Source: CAD feature listing. Evaluate the final solid. Frame: model axes, mm. A direction names the side the tool comes from. Round coordinates to 2 decimals unless told otherwise and drop trailing zeros. Write each loop counter-clockwise with the first axis right and the second up, starting at its lowest first coordinate (ties: lowest second). Pieces come first, ordered by that corner, then holes.
```python
from build123d import *

# Parameters (mm, degrees)
SKETCH_1_W          = 15
SKETCH_1_H          = 32
EXTRUDE_1_DEPTH     = 2
SKETCH_2_W          = 10
SKETCH_2_H          = 6
EXTRUDE_2_DEPTH     = 6
CHAMFER_1_SIZE      = 1
SKETCH_3_R          = 1.5
CUT_EXTRUDE_1_DEPTH = 28


with BuildPart() as part:
    # 草图1 → 凸台-拉伸1 (new body)
    with BuildSketch(Plane.XY):
        Rectangle(SKETCH_1_W, SKETCH_1_H)
    extrude(amount=EXTRUDE_1_DEPTH)

    # 草图2 → 凸台-拉伸2 (add)
    with BuildSketch(Plane(origin=(0, 0, 0), x_dir=(-1, 0, 0), z_dir=(0, 0, -1))):
        with Locations((0, 13)):
            Rectangle(SKETCH_2_W, SKETCH_2_H)
    extrude(amount=EXTRUDE_2_DEPTH)

    # 倒角1
    chamfer_1_edges = [part.edges().sort_by_distance(p)[0] for p in [
        (0, 10, -6),
        (-5, 13, -6),
        (0, 16, -6),
        (5, 13, -6),
    ]]
    chamfer(chamfer_1_edges, length=CHAMFER_1_SIZE)

    # 草图3 → 切除-拉伸1 (cut)
    with BuildSketch(Plane.XY.offset(2)):
        with Locations((0, -9)):
            Circle(SKETCH_3_R)
    extrude(amount=-CUT_EXTRUDE_1_DEPTH, mode=Mode.SUBTRACT)


solid = part.part
```
Q1. Pin query (flat end, axial travel): P1, Ø7.5, axis at x = -2.5, y = 0.5, coming from the -Z side; P2, Ø4, axis at y = 13, z = -2.5, coming from the +X side; P3, Ø4, axis at y = 12, z = -2.5, coming from the -X side. Return the tip coordinate at first contact, or that it passes through.
Q2. Section query D-D, the plane z = -3.75. Output: boundary loops of the cut face in (x, y).
Q3. Section query B-B, the plane y = -9. Output: boundary loops of the cut face in (x, z).
Q4. Mould query, pull axis X, two halves, no side actions, for faces 3 (the face through (-0.325, -10.464, 1.014)), 4 (the face through (-5, 13, -2)), 5 (the face through (5, 13, -2)), 6 (the face through (0.1, 15.5, -5.5)). Classes: pulls with the +X half, pulls with the -X half, needs draft (parallel to the pull), parting line crosses it, or undercut.
Q5. Section query C-C, the plane x = -2.5. Output: boundary loops of the cut face in (y, z).
Q6. Section query A-A, the plane x = 0. Output: boundary loops of the cut face in (y, z), and give its area (3 significant figures).
Q7. Line query: line 1 (Y direction, x = 0, z = 1); line 2 (Z direction, x = 2.5, y = -14); line 3 (Y direction, x = -1.75, z = -1.5). Output: solid intervals per line, ascending.
Q8. Set-up query: faces 1 (the face through (4.5, 13, -5.5)), 2 (the face through (0, 10, -2)). Return all of +Z, -Z, +X, -X, +Y, -Y with unobstructed straight access to the full face (end or side cutting, diameter ignored); none if empty.
Filled in:
1. P1: stops at z = 0
1. P2: stops at x = 5
1. P3: stops at x = -5
2. outline: (-5, 10) - (5, 10) - (5, 16) - (-5, 16) - close
3. outline: (-7.5, 0) - (-1.5, 0) - (-1.5, 2) - (-7.5, 2) - close; (1.5, 0) - (7.5, 0) - (7.5, 2) - (1.5, 2) - close
4. face 3: undercut
4. face 4: pulls with the -X half
4. face 5: pulls with the +X half
4. face 6: needs draft
5. outline: (-16, 0) - (10, 0) - (10, -5) - (11, -6) - (15, -6) - (16, -5) - (16, 2) - (-16, 2) - close
6. outline: (-16, 0) - (-10.5, 0) - (-10.5, 2) - (-16, 2) - close; (-7.5, 0) - (10, 0) - (10, -5) - (11, -6) - (15, -6) - (16, -5) - (16, 2) - (-7.5, 2) - close
6. area: 93.0 mm2
7. line 1: y = -16 to -10.5, -7.5 to 16
7. line 2: z = 0 to 2
7. line 3: y = 10 to 16
8. face 1: -Z, +X, +Y, -Y
8. face 2: -Z, +X, -X, -Y
